from build123d import *

# Parameters (mm, degrees)
SKETCH1_W           = 20
SKETCH1_H           = 8
BOSS_EXTRUDE1_DEPTH = 140
CUT_EXTRUDE1_DEPTH  = 141.584494166
BOSS_EXTRUDE2_DEPTH = 4
CUT_EXTRUDE2_DEPTH  = 142.393069137
BOSS_EXTRUDE3_DEPTH = 18
SKETCH7_W           = 16
SKETCH7_H           = 4
BOSS_EXTRUDE4_DEPTH = 40
SKETCH8_R           = 1.5
CUT_EXTRUDE3_DEPTH  = 141.712472795
SKETCH9_W           = 15
SKETCH9_H           = 30
CUT_EXTRUDE4_DEPTH  = 1.5
CUT_EXTRUDE5_DEPTH  = 2
SKETCH11_R          = 2.5
CUT_EXTRUDE6_DEPTH  = 142.50618361
SKETCH12_R          = 2.5
CUT_EXTRUDE7_DEPTH  = 142.05318146
SKETCH13_R          = 1.5
CUT_EXTRUDE8_DEPTH  = 15
SKETCH14_R          = 1.5
CUT_EXTRUDE9_DEPTH  = 15


with BuildPart() as part:
    # Sketch1 → Boss-Extrude1 (new body)
    with BuildSketch(Plane.XY):
        with Locations((0, 2)):
            Rectangle(SKETCH1_W, SKETCH1_H)
    extrude(amount=BOSS_EXTRUDE1_DEPTH)

    # Sketch2 → Cut-Extrude1 (cut, through all)
    with BuildSketch(Plane(origin=(0, 6, 0), x_dir=(1, 0, 0), z_dir=(0, 1, 0))):
        with BuildLine():
            Line((-10, 0), (-4, 0))
            Line((-4, 0), (-4, -98))
            ThreePointArc((-4, -98), (-5.757359313, -102.242640687), (-10, -104))
            Line((-10, -104), (-10, 0))
        make_face()
        with BuildLine():
            Line((10, -104), (10, 0))
            Line((10, 0), (4, 0))
            Line((4, 0), (4, -98))
            ThreePointArc((4, -98), (5.757359313, -102.242640687), (10, -104))
        make_face()
    extrude(amount=-CUT_EXTRUDE1_DEPTH, mode=Mode.SUBTRACT)

    # Sketch3 → Boss-Extrude2 (add, symmetric)
    with BuildSketch(Plane(origin=(0, 0, 0), x_dir=(0, 0, -1), z_dir=(1, 0, 0))):
        with BuildLine():
            Line((-140, 6), (0, 6))
            Line((0, 6), (0, 14))
            Line((0, 14), (-132, 14))
            ThreePointArc((-132, 14), (-137.656854249, 11.656854249), (-140, 6))
        make_face()
    extrude(amount=BOSS_EXTRUDE2_DEPTH, both=True)

    # Sketch4 → Cut-Extrude2 (cut, through all)
    with BuildSketch(Plane(origin=(4, 0, 0), x_dir=(0, 0, -1), z_dir=(1, 0, 0))):
        with BuildLine():
            Line((-35, -2), (-35, 2.95445115))
            ThreePointArc((-35, 2.95445115), (-36.045804216, 5.6512506), (-38.636363636, 6.937887932))
            ThreePointArc((-38.636363636, 6.937887932), (-47.636287443, 4.910736388), (-53.747727085, -2))
            Line((-53.747727085, -2), (-35, -2))
        make_face()
    extrude(amount=-CUT_EXTRUDE2_DEPTH, mode=Mode.SUBTRACT)

    # Sketch6 → Boss-Extrude3 (add)
    with BuildSketch(Plane(origin=(0, 14, 0), x_dir=(1, 0, 0), z_dir=(0, 1, 0))):
        with BuildLine():
            Line((-4, 0), (-8, 0))
            Line((-8, 0), (-8, -31))
            ThreePointArc((-8, -31), (-5.171572875, -32.171572875), (-4, -35))
            Line((-4, -35), (4, -35))
            ThreePointArc((4, -35), (5.171572875, -32.171572875), (8, -31))
            Line((8, -31), (8, 0))
            Line((8, 0), (4, 0))
            Line((4, 0), (-4, 0))
        make_face()
    extrude(amount=-BOSS_EXTRUDE3_DEPTH)

    # Sketch7 → Boss-Extrude4 (add)
    with BuildSketch(Plane(origin=(0, 0, 0), x_dir=(-1, 0, 0), z_dir=(0, 0, -1))):
        with Locations((0, -2)):
            Rectangle(SKETCH7_W, SKETCH7_H)
    extrude(amount=BOSS_EXTRUDE4_DEPTH)

    # Sketch8 → Cut-Extrude3 (cut, through all)
    with BuildSketch(Plane(origin=(0, 6, 0), x_dir=(1, 0, 0), z_dir=(0, 1, 0))):
        with Locations(Location((7.5, -137, 0), (0, 0, 270))):
            Circle(SKETCH8_R)
        with Locations(Location((7.5, -107, 0), (0, 0, 270))):
            Circle(SKETCH8_R)
        with Locations(Location((-7.5, -107, 0), (0, 0, 180))):
            Circle(SKETCH8_R)
        with Locations(Location((-7.5, -137, 0), (0, 0, 180))):
            Circle(SKETCH8_R)
    extrude(amount=-CUT_EXTRUDE3_DEPTH, mode=Mode.SUBTRACT)

    # Sketch9 → Cut-Extrude4 (cut)
    with BuildSketch(Plane.XZ.offset(2)):
        with Locations((0, 122)):
            Rectangle(SKETCH9_W, SKETCH9_H)
    extrude(amount=-CUT_EXTRUDE4_DEPTH, mode=Mode.SUBTRACT)

    # Sketch10 → Cut-Extrude5 (cut)
    with BuildSketch(Plane.XZ.offset(2)):
        with BuildLine():
            Line((3, 79), (3, 65))
            ThreePointArc((3, 65), (0, 62), (-3, 65))
            Line((-3, 65), (-3, 79))
            ThreePointArc((-3, 79), (0, 82), (3, 79))
        make_face()
    extrude(amount=-CUT_EXTRUDE5_DEPTH, mode=Mode.SUBTRACT)

    # Sketch11 → Cut-Extrude6 (cut, through all)
    with BuildSketch(Plane(origin=(0, 14, 0), x_dir=(1, 0, 0), z_dir=(0, 1, 0))):
        with Locations(Location((0, -26, 0), (0, 0, 270))):
            Circle(SKETCH11_R)
        with Locations(Location((0, -6, 0), (0, 0, 270))):
            Circle(SKETCH11_R)
    extrude(amount=-CUT_EXTRUDE6_DEPTH, mode=Mode.SUBTRACT)

    # Sketch12 → Cut-Extrude7 (cut, through all)
    with BuildSketch(Plane(origin=(0, 0, 0), x_dir=(1, 0, 0), z_dir=(0, 1, 0))):
        with Locations(Location((0, 10, 0), (0, 0, 270))):
            Circle(SKETCH12_R)
        with Locations(Location((0, 30, 0), (0, 0, 270))):
            Circle(SKETCH12_R)
    extrude(amount=-CUT_EXTRUDE7_DEPTH, mode=Mode.SUBTRACT)

    # Sketch13 → Cut-Extrude8 (cut)
    with BuildSketch(Plane(origin=(10, 0, 0), x_dir=(0, 0, -1), z_dir=(1, 0, 0))):
        with Locations((-119.9, 2)):
            Circle(SKETCH13_R)
    extrude(amount=-CUT_EXTRUDE8_DEPTH, mode=Mode.SUBTRACT)

    # Sketch14 → Cut-Extrude9 (cut)
    with BuildSketch(Plane(origin=(8, 0, 0), x_dir=(0, 0, -1), z_dir=(1, 0, 0))):
        with Locations((-10.9, 2)):
            Circle(SKETCH14_R)
    extrude(amount=-CUT_EXTRUDE9_DEPTH, mode=Mode.SUBTRACT)


solid = part.part
Verification items for the finished model (mm, model axes). A direction names the side the tool comes from. Give positions to 0.01 mm unless a question says otherwise; leave off trailing zeros. Write each loop counter-clockwise with the first axis right and the second up, starting at its lowest first coordinate (ties: lowest second). Pieces come first, ordered by that corner, then holes. Notation, with made-up numbers: M -33.75,26.25 L 9.25,26.25 A13 ccw 9.25,39.25 Z; hole C -16.5,71 d9. An arc over 180 degrees is marked long. Use CSV: the item, a comma, the result in double quotes.
1) Access from +Z, -Z, +X, -X, +Y, -Y to the whole of each face (thin tool, end or side, straight path). Record for faces 1 (the face through (0, -1, 62)), 2 (the face through (-1, -2, 100)), 3 (the face through (0, 7, 0)), 4 (the face through (-4, 8, 88)), 5 (the face through (4, 8, 88)).
Final values:
face 1,"-Y"
face 2,"+Z, +X, -X, -Y"
face 3,"-Z, +X, -X, +Y"
face 4,"-X, +Y"
face 5,"+X, +Y"
2) Cross-section at D-D (z = -10). Enter the section's corners in (x, y), plus the area to 3 significant figures.
Final values:
outline,"M -8,-4 L -2.5,-4 L -2.5,0 L -8,0 Z; M 2.5,-4 L 8,-4 L 8,0 L 2.5,0 Z"
area,"44.0 mm²"
3) Release check for a two-part mould opening along Y. For faces 6 (the face through (0, 0, -20)), 7 (the face through (2.61, 2.45, 118.47)), 8 (the face through (0.1, 5.1, 23.5)), 9 (the face through (-7, 2, 11)) record: released by +Y, released by -Y, zero draft, split by the parting line, or undercut.
Final values:
face 6,"released by +Y"
face 7,"undercut"
face 8,"zero draft"
face 9,"undercut"
4) Cross-section at C-C (z = 119.9). Enter the section's corners in (x, y), plus the area to 4 significant figures.
Final values:
outline,"M -10,-2 L -7.5,-2 L -7.5,-0.5 L 7.5,-0.5 L 7.5,-2 L 10,-2 L 10,0.5 L -5,0.5 L -5,3.5 L 10,3.5 L 10,6 L 4,6 L 4,14 L -4,14 L -4,6 L -10,6 Z"
area,"156.5 mm²"
5) Cross-section at B-B (y = 9). Enter the section's corners in (x, z), plus the area to 3 significant figures.
Final values:
outline,"M -8,0 L 8,0 L 8,31 A4 cw 4,35 L 4,139.42 L -4,139.42 L -4,35 A4 cw -8,31 Z; hole C 0,6 d5; hole C 0,26 d5"
area,"1,330 mm²"
6) Go/stop test with flat-tipped pins: pin 1 Ø10 at (x, y) = (-7.5, 12) entering from -Z; pin 2 Ø10 at (x, z) = (-3, 89.5) entering from -Y; pin 3 Ø10 at (x, z) = (7.5, 48.5) entering from -Y. Record where each tip stops, or that it passes through.
Final values:
pin 1,"z = 0"
pin 2,"y = -2"
pin 3,"y = 0.9"
7) Cross-section at A-A (z = 26). Enter the section's corners in (x, y).
Final values:
outline,"M -8,-4 L -2.5,-4 L -2.5,14 L -8,14 Z; M 2.5,-4 L 8,-4 L 8,14 L 2.5,14 Z"
8) Material ranges on line 1 along X through (y, z) = (2.5, 137); line 2 along X through (y, z) = (-2.3, -30); line 3 along Y through (x, z) = (4.5, 10.9), recorded low to high.
Final values:
line 1,"-10 to -9, -6 to 6, 9 to 10"
line 2,"-8 to -2.5, 2.5 to 8"
line 3,"-4 to 0.5, 3.5 to 14"
